Source: CAD feature listing. Evaluate the final solid. Frame: model axes, mm. Round coordinates to 2 decimals unless told otherwise and drop trailing zeros. Write each loop counter-clockwise with the first axis right and the second up, starting at its lowest first coordinate (ties: lowest second). Pieces come first, ordered by that corner, then holes. Notation, with made-up numbers: M 53,-18 L 85,-18 A21 ccw 85,14 Z; hole C 5,35 d4. An arc over 180 degrees is marked long. Answer in a Markdown table with one row per item.
from build123d import *
from build123d.topology import SkipClean

# Parameters (mm, degrees)
BASPROSKE_W       = 5
BASPROSKE_H       = 3
TOOTHCUT_DEPTH    = 7.557438524
TEETHCUTS_COUNT   = 10
TEETHCUTS_ANGLE   = 324
HUBNEARBOTH_START = 12.5000254
HUBNEABOTSKE_R    = 1.874
HUBNEARBOTH_DEPTH = 12.5000254
HUBFARSKE_R       = 1.874
HUBFAR_DEPTH      = 12.5000254
BORSKE_R          = 0.4
BORE_DEPTH        = 30.0000508


with BuildPart() as part:
    # BasProSke → Base-Revolve (revolve)
    with BuildSketch(Plane(origin=(0, 0, 0), x_dir=(1, 0, 0), z_dir=(0, 1, 0)), mode=Mode.PRIVATE) as base_revolve_sk:
        with Locations((2.5, 1.5)):
            Rectangle(BASPROSKE_W, BASPROSKE_H)
    revolve(base_revolve_sk.sketch.rotate(Axis((-10, 0, 0), (1, 0, 0)), 180), axis=Axis((-10, 0, 0), (1, 0, 0)))

    # TooCutSke → ToothCut (cut, through all)
    with BuildSketch(Plane(origin=(0, 0, 0), x_dir=(0, 0, -1), z_dir=(1, 0, 0))):
        with BuildLine():
            ThreePointArc((0.296449938, 1.850403587), (0, 1.874), (-0.296449938, 1.850403587))
            ThreePointArc((-0.296449938, 1.850403587), (-0.428089565, 2.470295585), (-0.905889751, 2.886591228))
            ThreePointArc((-0.905889751, 2.886591228), (0, 3.0254), (0.905889751, 2.886591228))
            ThreePointArc((0.905889751, 2.886591228), (0.428089565, 2.470295585), (0.296449938, 1.850403587))
        make_face()
    toothcut = extrude(amount=TOOTHCUT_DEPTH, mode=Mode.SUBTRACT)

    # TeethCuts: ToothCut ×10 about axis
    teethcuts_axis = Axis((-10, 0, 0), (1, 0, 0))
    for i in range(1, TEETHCUTS_COUNT):
        add(toothcut.rotate(teethcuts_axis, i * TEETHCUTS_ANGLE / (TEETHCUTS_COUNT - 1)), mode=Mode.SUBTRACT)

    # HubNeaBotSke → HubNearBoth (add)
    with SkipClean():  # the faces are left unmerged after this step: merging them gives an invalid solid
        with BuildSketch(Plane.ZY.offset(HUBNEARBOTH_START)):
            Circle(HUBNEABOTSKE_R)
        extrude(amount=-HUBNEARBOTH_DEPTH)

    # HubFarSke → HubFar (add)
    with SkipClean():  # the faces are left unmerged after this step: merging them gives an invalid solid
        with BuildSketch(Plane(origin=(5, 0, 0), x_dir=(0, 0, -1), z_dir=(1, 0, 0))):
            with Locations(Location((0, 0, 0), (0, 0, 180))):
                Circle(HUBFARSKE_R)
        extrude(amount=HUBFAR_DEPTH)

    # BorSke → Bore (cut, symmetric)
    with SkipClean():  # the faces are left unmerged after this step: merging them gives an invalid solid
        with BuildSketch(Plane(origin=(0, 0, 0), x_dir=(0, 0, -1), z_dir=(1, 0, 0))):
            with Locations(Location((0, 0, 0), (0, 0, 180))):
                Circle(BORSKE_R)
        extrude(amount=BORE_DEPTH, both=True, mode=Mode.SUBTRACT)


solid = part.part
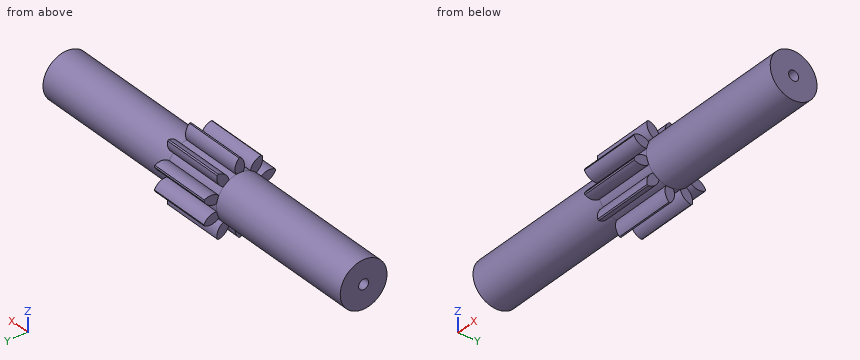
Q1. Contact query for flat-ended pins moving along their axis: pin 1 Ø0.6 at (y, z) = (0, 2.5) entering from +X; pin 2 Ø3 at (x, y) = (-6, -1) entering from +Z; pin 3 Ø0.8 at (y, z) = (1.5, 2) entering from -X. Output: stop coordinate, or through.
Solutions:
| item | result |
|---|---|
| pin 1 | stops at x = 5 |
| pin 2 | stops at z = 1.87 |
| pin 3 | stops at x = 0 |
Q2. Section B-B (y = -2.35). Return loops of the section in (x, z).
Solutions:
| item | result |
|---|---|
| outline | M 0,-1.11 L 5,-1.11 L 5,-0.37 L 0,-0.37 Z; M 0,0.37 L 5,0.37 L 5,1.11 L 0,1.11 Z |
Q3. Section C-C (x = 16). Return loops of the section in (y, z), and give its area (3 significant figures).
Solutions:
| item | result |
|---|---|
| outline | C 0,0 d3.75; hole C 0,0 d0.8 |
| area | 10.5 mm2 |
Q4. Section A-A (z = 0). Return loops of the section in (x, y).
Solutions:
| item | result |
|---|---|
| outline | M -12.5,-1.87 L 17.5,-1.87 L 17.5,-0.4 L -12.5,-0.4 Z; M -12.5,0.4 L 17.5,0.4 L 17.5,1.87 L -12.5,1.87 Z |
Q5. Material intervals for probe 1 along Y at (x, z) = (4.5, 0); probe 2 along Y at (x, z) = (4.5, 2.3), sorted ascending.
Solutions:
| item | result |
|---|---|
| probe 1 | y = -1.87 to -0.4, 0.4 to 1.87 |
| probe 2 | y = -1.82 to -1.28, -0.38 to 0.38, 1.28 to 1.82 |
